Could you check a few things on this model? Use its own coordinates, in mm. A direction names the side the tool comes from. Round coordinates to 2 decimals unless told otherwise and drop trailing zeros. Loops run counter-clockwise (first coordinate to the right, second up) from the corner with the lowest first, then second, coordinate; pieces in that order, holes last. Notation, with made-up numbers: (-24, 87) - (19, 87) arc R15 ccw to (19, 108) - close; hole circle Ø3 at (2, 86). An arc over 180 degrees is marked (long way). Use one line per item in the form item = value.
```python
from build123d import *

# Parameters (mm, degrees)
SKETCH1_W           = 25.4
SKETCH1_H           = 25.4
BOSS_EXTRUDE1_DEPTH = 342.9
SKETCH2_W           = 22.098
SKETCH2_H           = 22.098
CUT_EXTRUDE1_DEPTH  = 357.529874987
SKETCH4_R           = 3.175
CUT_EXTRUDE3_DEPTH  = 354.770733702


with BuildPart() as part:
    # Sketch1 → Boss-Extrude1 (new body)
    with BuildSketch(Plane.XY):
        with Locations((-70.535581478, -38.339002092)):
            Rectangle(SKETCH1_W, SKETCH1_H)
    extrude(amount=BOSS_EXTRUDE1_DEPTH)

    # Sketch2 → Cut-Extrude1 (cut, through all)
    with BuildSketch(Plane.XY.offset(342.9)):
        with Locations((-70.535581478, -38.339002092)):
            Rectangle(SKETCH2_W, SKETCH2_H)
    extrude(amount=-CUT_EXTRUDE1_DEPTH, mode=Mode.SUBTRACT)

    # Sketch4 → Cut-Extrude3 (cut, through all)
    with BuildSketch(Plane.XZ.offset(51.039002092)):
        with Locations(Location((-70.535581478, 330.2, 0), (0, 0, 270))):
            Circle(SKETCH4_R)
    extrude(amount=-CUT_EXTRUDE3_DEPTH, mode=Mode.SUBTRACT)


solid = part.part
```
1. We'd pull the mould along Y, two halves only. Please class faces 1 (the face through (-71, -49.388, 174)), 2 (the face through (-71, -25.639, 169)), 3 (the face through (-71, -51.039, 169)): +Y half, -Y half, draft (parallel to the pull), parting line (faces both ways), or undercut.
Solution:
face_1 = undercut
face_2 = +Y half
face_3 = -Y half
2. Please list where these lines run through material, in increasing order: line 1 along X through (y, z) = (-33.75, 289.5); line 2 along X through (y, z) = (-26.05, 330.2); line 3 along Y through (x, z) = (-60, 257.5).
Solution:
line_1 = -83.24 to -81.58, -59.49 to -57.84
line_2 = -83.24 to -73.71, -67.36 to -57.84
line_3 = -51.04 to -49.39, -27.29 to -25.64
3. If we section it at C-C, the plane z = 330.2: Write out the boundary of the cut face in (x, y).
Solution:
outline = (-83.24, -51.04) - (-73.71, -51.04) - (-73.71, -49.39) - (-81.58, -49.39) - (-81.58, -27.29) - (-73.71, -27.29) - (-73.71, -25.64) - (-83.24, -25.64) - close; (-67.36, -51.04) - (-57.84, -51.04) - (-57.84, -25.64) - (-67.36, -25.64) - (-67.36, -27.29) - (-59.49, -27.29) - (-59.49, -49.39) - (-67.36, -49.39) - close
4. If we section it at B-B, the plane z = 160.5: Write out the boundary of the cut face in (x, y).
Solution:
outline = (-83.24, -51.04) - (-57.84, -51.04) - (-57.84, -25.64) - (-83.24, -25.64) - close; hole (-81.58, -49.39) - (-59.49, -49.39) - (-59.49, -27.29) - (-81.58, -27.29) - close
5. If we section it at A-A, the plane x = -78.5: Write out the boundary of the cut face in (y, z).
Solution:
outline = (-51.04, 0) - (-49.39, 0) - (-49.39, 342.9) - (-51.04, 342.9) - close; (-27.29, 0) - (-25.64, 0) - (-25.64, 342.9) - (-27.29, 342.9) - close
6. On a 3-axis mill with a long thin cutter (end or side, diameter ignored), from which of +Z, -Z, +X, -X, +Y, -Y can I reach the whole of each face in a straight line? I mean faces 4 (the face through (-81.585, -38, 174)), 5 (the face through (-68.39, -26.48, 332.54)). Say none if no direction works.
Solution:
face_4 = +Z, -Z
face_5 = +Y, -Y
